from build123d import *

# Parameters (mm, degrees)
SKETCH1_W           = 76.595992709
SKETCH1_H           = 226.770325479
SKETCH1_W_2         = 125.310344828
SKETCH1_H_2         = 58.689655172
SKETCH1_W_3         = 80.103448276
SKETCH1_H_3         = 230
BOSS_EXTRUDE1_DEPTH = 130
SKETCH3_W           = 109.68672873
SKETCH3_H           = 20.160489082
CUT_EXTRUDE1_DEPTH  = 100
SKETCH7_W           = 108.256911282
SKETCH7_H           = 50
CUT_EXTRUDE3_DEPTH  = 40


with BuildPart() as part:
    # Sketch1 → Boss-Extrude1 (new body)
    with BuildSketch(Plane.XY):
        with Locations((-163.608341182, -20.592059291)):
            Rectangle(SKETCH1_W, SKETCH1_H)
        with Locations((-62.655172414, 63.448275862)):
            Rectangle(SKETCH1_W_2, SKETCH1_H_2)
        with Locations((40.051724138, -22.206896552)):
            Rectangle(SKETCH1_W_3, SKETCH1_H_3)
    extrude(amount=BOSS_EXTRUDE1_DEPTH)

    # Sketch3 → Cut-Extrude1 (cut)
    with BuildSketch(Plane.XY.offset(130)):
        with Locations((-62.780812257, 65.439975471)):
            Rectangle(SKETCH3_W, SKETCH3_H)
    extrude(amount=-CUT_EXTRUDE1_DEPTH, mode=Mode.SUBTRACT)

    # Sketch7 → Cut-Extrude3 (cut)
    with BuildSketch(Plane(origin=(0, 34.103448276, 0), x_dir=(-1, 0, 0), z_dir=(0, -1, 0))):
        with Locations((63.495720981, -64.04122146)):
            Rectangle(SKETCH7_W, SKETCH7_H)
    extrude(amount=-CUT_EXTRUDE3_DEPTH, mode=Mode.SUBTRACT)


solid = part.part
CAD build for the part. Positions are in the model's coordinates, mm. A direction names the side the tool comes from. Give positions to 0.01 mm unless a question says otherwise; leave off trailing zeros. Write each loop counter-clockwise with the first axis right and the second up, starting at its lowest first coordinate (ties: lowest second). Pieces come first, ordered by that corner, then holes. Notation, with made-up numbers: M -32,38 L -13,38 A5 ccw -13,42 Z; hole C 17,34 d9. An arc over 180 degrees is marked long. Put each result on its own line as item: value. Start each with the question number.
(1) Probe L1, parallel to X at y = -71, z = 69.5; L2, parallel to Z at x = -50, y = 52; L3, parallel to X at y = 63, z = 111.5. List the from-to ranges inside material, lowest first.
(2) Band-saw the part on D-D, the plane z = 81. Write the cut outline in (x, y).
(3) Mould opens along Z. For faces 6 (the face through (-164, -133.977, 64)), 7 (the face through (-63, 45, 89.041)), 8 (the face through (-126, 5, 0)) say: +Z half, -Z half, draft (parallel to the pull), parting line (faces both ways), or undercut.
(4) Flat gauge pins, fed straight in: pin 1 Ø6.5 at (x, y) = (-62.5, 39.5) entering from -Z; pin 2 Ø23 at (x, z) = (-162.5, 85.5) entering from -Y; pin 3 Ø10 at (x, z) = (-41, 17.5) entering from -Y; pin 4 Ø2 at (x, z) = (-14, 58.5) entering from -Y. Where does each tip first touch, or does it go through?
(5) Band-saw the part on B-B, the plane y = -51.5. Write the cut outline in (x, z), and give its area (3 significant figures).
(6) Band-saw the part on A-A, the plane z = 101. Write the cut outline in (x, y).
(7) Band-saw the part on C-C, the plane x = -83. Write the cut outline in (y, z), and give its area (3 significant figures).
(8) Which spindle directions (+Z, -Z, +X, -X, +Y, -Y) get a long thin tool onto all of the face, cutting with end or side? Do faces 1 (the face through (-117.624, 59, 70)), 2 (the face through (39, -137.207, 64)), 3 (the face through (-125.31, -51, 64)), 4 (the face through (-9.367, 45, 64)), 5 (the face through (-7.937, 65, 81)). Say none if no direction does.
Response values:
1. L1: x = -201.91 to -125.31, 0 to 80.1
1. L2: z = 0 to 39.04, 89.04 to 130
1. L3: x = -201.91 to -117.62, -7.94 to 80.1
2. outline: M -201.91,-133.98 L -125.31,-133.98 L -125.31,34.1 L -117.62,34.1 L -117.62,75.52 L -7.94,75.52 L -7.94,55.36 L -9.37,55.36 L -9.37,34.1 L 0,34.1 L 0,-137.21 L 80.1,-137.21 L 80.1,92.79 L -201.91,92.79 Z
3. face 6: draft
3. face 7: undercut
3. face 8: -Z half
4. pin 1: stops at z = 0
4. pin 2: stops at y = -133.98
4. pin 3: stops at y = 34.1
4. pin 4: stops at y = 75.52
5. outline: M -201.91,0 L -125.31,0 L -125.31,130 L -201.91,130 Z; M 0,0 L 80.1,0 L 80.1,130 L 0,130 Z
5. area: 20,400 mm2
6. outline: M -201.91,-133.98 L -125.31,-133.98 L -125.31,34.1 L 0,34.1 L 0,-137.21 L 80.1,-137.21 L 80.1,92.79 L -201.91,92.79 Z; hole M -117.62,55.36 L -7.94,55.36 L -7.94,75.52 L -117.62,75.52 Z
7. outline: M 34.1,0 L 92.79,0 L 92.79,130 L 75.52,130 L 75.52,30 L 55.36,30 L 55.36,39.04 L 34.1,39.04 Z; M 34.1,89.04 L 55.36,89.04 L 55.36,130 L 34.1,130 Z
7. area: 4,550 mm2
8. face 1: none
8. face 2: +Z, -Z, +X, -X, -Y
8. face 3: +Z, -Z, -Y
8. face 4: -Y
8. face 5: +Z
